Build history of the part. All positions in model axes, mm. Coordinates: 2 decimals unless noted, no trailing zeros. Order: outer loops, then holes, each group sorted by start corner. A loop starts at its lowest first (then second) coordinate and runs counter-clockwise, first axis right, second up. Notation, with made-up numbers: (76.5, -17) - (87.5, -17) arc R19 ccw to (87.5, -5) - close; hole circle Ø3 at (-3.5, 81.25). An arc over 180 degrees is marked (long way). Return JSON: item names as keys, results as strings.
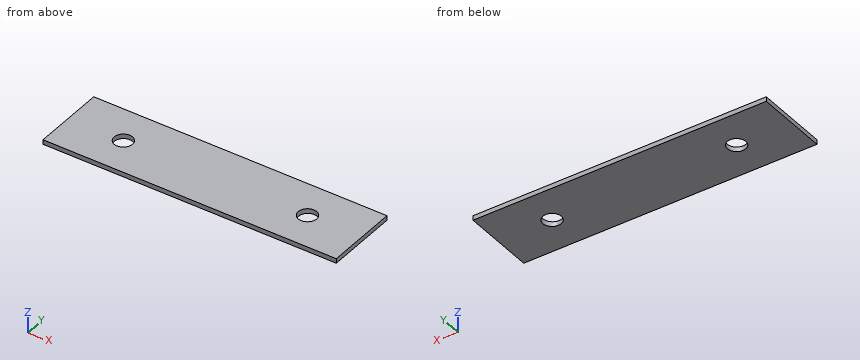
Autodesk Inventor part; units mm, degrees
ref_plane "Work Plane2" through (117.4846, -2.3812, 5.6317) normal (-0.0842, 0, 0.9965) x (0, 1, 0)
ref_plane "YZ Plane" through (0, 0, 0) normal (1, 0, 0) x (0, 1, 0)
ref_plane "XZ Plane" through (0, 0, 0) normal (0, 1, 0) x (-1, 0, 0)
sketch "Sketch1" plane through (0, 0, 0) normal (0, 0, 1) x (1, 0, 0)
  line L0 (0, 0) -> (50.8, 0)
  line L1 (50.8, 0) -> (50.8, 12.7)
  line L2 (50.8, 12.7) -> (0, 12.7)
  line L3 (0, 12.7) -> (0, 0)
  line L4 (25.4, 12.7) -> (25.4, 0) construction
  line L5 (9.525, 6.35) -> (41.275, 6.35) construction
  circle A0 centre (9.525, 6.35) radius 1.5875
  circle A1 centre (41.275, 6.35) radius 1.5875
  point P0 (25.4, 6.35)
  dimension "d0" = 12.7
  dimension "d1" = 50.8
  dimension "d2" = 3.175
  dimension "d3" = 9.525
extrude "Extrusion1" add sketch "Sketch1" along normal blind 0.7937 contours L3 L2 L1 L0 | A1
ref_plane "Work Plane2" through (117.4846, -2.3812, 5.6317) normal (-0.0842, 0, 0.9965) x (0, 1, 0)
sketch "Sketch2" plane through (117.4846, -2.3812, 5.6317) normal (-0.0842, 0, 0.9965) x (0, 1, 0)
  circle A0 centre (8.7312, 76.2) radius 1.5875
  line L0 (18.2562, 0) -> (0, 0) construction
  line L1 (18.2562, 0) -> (18.2562, 92.075) construction
  line L2 (0, 92.075) -> (18.2562, 92.075) construction
  line L3 (0, 0) -> (0, 92.075) construction
  point P0 (2.3812, 117.5418)
extrude "Extrusion2" cut sketch "Sketch2" along normal through all
properties part number "Hopper Bracing P12 to P1" material "Aluminum 6061"
1. Cut at A-A on y = 6.35. Give the cut face in (x, z), plus the area to 3 significant figures.
Check values:
{"outline": "(0, 0) - (7.94, 0) - (7.94, 0.79) - (0, 0.79) - close; (11.11, 0) - (39.9, 0) - (39.83, 0.79) - (11.11, 0.79) - close; (43.02, 0.79) - (43.08, 0) - (50.8, 0) - (50.8, 0.79) - close", "area": "35.3 mm²"}
2. Drop flat-ended pins along their axis: pin 1 (3 mm diameter, centred on x = 9.525, y = 6.35, fed in from +Z); pin 2 (2 mm diameter, centred on x = 9.5, y = 5.5, fed in from -Z). Give the stop position or say it passes through.
Check values:
{"pin 1": "through", "pin 2": "z = 0"}
3. Probe L1, parallel to X at y = 5.25, z = 0.2; L2, parallel to X at y = 5.5, z = 0.45; L3, parallel to Y at x = 10.5, z = 0.75. List the from-to ranges inside material, lowest first.
Check values:
{"L1": "0 to 8.38, 10.67 to 40.32, 42.62 to 50.8", "L2": "0 to 8.18, 10.87 to 40.11, 42.8 to 50.8", "L3": "0 to 5.1, 7.6 to 12.7"}
4. Cut at B-B on z = 0.6. State how many separate pieces and enclosed holes the cut face has, plus the area to 3 significant figures.
Check values:
{"separate pieces": "1", "enclosed holes": "2", "area": "629 mm²"}
